Autodesk Inventor part; units mm, degrees
ref_plane "YZ Plane" through (0, 0, 0) normal (1, 0, 0) x (0, 1, 0)
ref_plane "XZ Plane" through (0, 0, 0) normal (0, 1, 0) x (-1, 0, 0)
ref_plane "XY Plane" through (0, 0, 0) normal (0, 0, 1) x (1, 0, 0)
sketch "Sketch1" plane through (0, 0, 0) normal (0, 0, 1) x (1, 0, 0)
  line L0 (-110, 70) -> (110, 70) construction
  line L1 (110, 70) -> (110, -70) construction
  line L2 (110, -70) -> (-110, -70) construction
  line L3 (-110, -70) -> (-110, 70) construction
  circle A0 centre (-90, 55) radius 5
  circle A1 centre (-90, -55) radius 5
  circle A2 centre (90, -55) radius 5
  circle A3 centre (-10, 45) radius 5
  line L4 (-67, 0) -> (-42, 0) construction
  line L5 (-42, 0) -> (-42, -30) construction
  line L6 (-42, -30) -> (-67, -30) construction
  line L7 (-67, -30) -> (-67, 0) construction
  circle A4 centre (-54.5, -11) radius 10 construction
  circle A5 centre (-63.5044, -24.4163) radius 3 construction
  circle A6 centre (-57.3559, -26.4695) radius 3 construction
  circle A7 centre (-51.263, -24.6531) radius 3 construction
  circle A8 centre (-45.3418, -26.5938) radius 3 construction
  arc A9 (-80.6122, 51.5548) -> (-99.3921, 51.5667) centre (-90, 55) ccw
  arc A10 (0, 45) -> (-16.4942, 52.6043) centre (-10, 45) ccw
  arc A11 (89.2256, -64.97) -> (88.3846, -45.1313) centre (90, -55) ccw
  line L8 (-100, 55) -> (-93.7227, 20.2343) construction
  line L9 (-93.7227, 20.2343) -> (-93.7227, 2.3339) construction
  line L10 (-93.7227, 2.3339) -> (-93.7227, -15.5707) construction
  line L11 (-93.7227, -15.5707) -> (-100, -55) construction
  spline S0 degree 4 poles (-100, 55) (-93.7227, 20.2343) (-93.7227, 2.3339) (-93.7227, -15.5707) (-100, -55) knots 1 1 1 1 1 2 2 2 2 2
  line L12 (-80, 55.0121) -> (-83.1179, 37.7603) construction
  line L13 (-33.0458, 38.469) -> (-16.4942, 52.6043) construction
  spline S1 degree 3 poles (-81.8662, -0.1941) (-57.8765, 11.5233) (-33.0458, 38.469) (-16.4942, 52.6043) knots 1.047287 1.047287 1.047287 1.047287 2 2 2 2
  line L14 (66.7614, -48.6708) -> (88.3846, -45.1313) construction
  line L15 (-90, -65) -> (-39.6885, -60.8902) construction
  line L16 (-39.6885, -60.8902) -> (0, -60.8902) construction
  line L17 (0, -60.8902) -> (36.6975, -60.8902) construction
  line L18 (36.6975, -60.8902) -> (89.2256, -64.97) construction
  spline S2 degree 4 poles (-90, -65) (-39.6885, -60.8902) (0, -60.8902) (36.6975, -60.8902) (89.2256, -64.97) knots 1 1 1 1 1 2 2 2 2 2
  spline S3 degree 3 poles (-13.6002, 30.0827) (-5.3402, 7.268) (-5.6398, -29.8026) (-10.5938, -50.667) knots 1.109736 1.109736 1.109736 1.109736 1.972131 1.972131 1.972131 1.972131
  line L19 (0, 45) -> (0, 17.1156) construction
  spline S4 degree 3 poles (0, 45) (0, 17.1156) (4.0635, -28.5965) (11.4843, -50.8799) knots 1 1 1 1 1.973632 1.973632 1.973632 1.973632
  arc A12 (-99.5185, -51.9345) -> (-88.3922, -64.8699) centre (-90, -55) ccw
  spline S5 degree 3 poles (-82.1602, -33.4696) (-73.7302, -5.1617) (-50.5606, 15.5541) (-16.7734, 31.5924) knots 1.116691 1.116691 1.116691 1.116691 1.939936 1.939936 1.939936 1.939936
  line L20 (-82.1602, -33.4696) -> (-73.7302, -5.1617) construction
  spline S6 degree 4 poles (-80, 55.0121) (-83.1179, 37.7603) (-84.6762, 24.5857) (-85.4554, 13.4176) (-85.4634, 2.054) knots 1 1 1 1 1 1.500456 1.500456 1.500456 1.500456 1.500456
  spline S7 degree 4 poles (-82.1602, -33.4696) (-82.7141, -35.9408) (-82.3572, -38.6467) (-81.9633, -41.4647) (-81.5291, -44.4067) knots 1.850189 1.850189 1.850189 1.850189 1.850189 1.936877 1.936877 1.936877 1.936877 1.936877
  line L21 (-82.1602, -33.4696) -> (-82.7141, -35.9408) construction
  spline S8 degree 4 poles (-79.5204, -46.4981) (-59.8812, -49.3583) (-42.9543, -51.1251) (-27.6277, -52.1691) (-12.9522, -52.5883) knots 1.043038 1.043038 1.043038 1.043038 1.043038 1.405573 1.405573 1.405573 1.405573 1.405573
  spline S9 degree 4 poles (13.9278, -52.5889) (30.7931, -52.1056) (47.9331, -50.8127) (66.7614, -48.6708) (88.3846, -45.1313) knots 1.574481 1.574481 1.574481 1.574481 1.574481 2 2 2 2 2
  arc A13 (-13.6002, 30.0827) -> (-16.7734, 31.5924) centre (-15.9509, 29.2316) ccw
  line L22 (-73.7302, -5.1617) -> (-50.5606, 15.5541) construction
  line L23 (-50.5606, 15.5541) -> (-16.7734, 31.5924) construction
  line L24 (-13.6002, 30.0827) -> (-5.3402, 7.268) construction
  arc A14 (-13.2443, -52.5799) -> (-10.5938, -50.667) centre (-13.0262, -50.0894) ccw
  line L25 (-5.3402, 7.268) -> (-5.6398, -29.8026) construction
  line L26 (-5.6398, -29.8026) -> (-10.5938, -50.667) construction
  line L27 (-27.6277, -52.1691) -> (-12.9522, -52.5883) construction
  arc A15 (11.4843, -50.8799) -> (13.9278, -52.5889) centre (13.8562, -50.09) ccw
  line L28 (0, 17.1156) -> (4.0635, -28.5965) construction
  line L29 (4.0635, -28.5965) -> (11.4843, -50.8799) construction
  line L30 (13.9278, -52.5889) -> (30.7931, -52.1056) construction
  line L31 (30.7931, -52.1056) -> (47.9331, -50.8127) construction
  line L32 (47.9331, -50.8127) -> (66.7614, -48.6708) construction
  arc A16 (-81.5291, -44.4067) -> (-79.5204, -46.4981) centre (-79.0558, -44.0416) ccw
  line L33 (-82.7141, -35.9408) -> (-82.3572, -38.6467) construction
  line L34 (-82.3572, -38.6467) -> (-81.9633, -41.4647) construction
  line L35 (-81.9633, -41.4647) -> (-81.5291, -44.4067) construction
  line L36 (-79.5204, -46.4981) -> (-59.8812, -49.3583) construction
  line L37 (-59.8812, -49.3583) -> (-42.9543, -51.1251) construction
  line L38 (-42.9543, -51.1251) -> (-27.6277, -52.1691) construction
  arc A17 (-85.4634, 2.054) -> (-81.8662, -0.1941) centre (-82.9634, 2.0522) ccw
  line L39 (-83.1179, 37.7603) -> (-84.6762, 24.5857) construction
  line L40 (-84.6762, 24.5857) -> (-85.4554, 13.4176) construction
  line L41 (-85.4554, 13.4176) -> (-85.4634, 2.054) construction
  line L42 (-81.8662, -0.1941) -> (-57.8765, 11.5233) construction
  line L43 (-57.8765, 11.5233) -> (-33.0458, 38.469) construction
  point P0 (0, 0)
  dimension "d1" = 70
  dimension "d2" = 70
  dimension "d3" = 110
  dimension "d4" = 110
  dimension "d5" = 10
  dimension "d6" = 10
  dimension "d7" = 10
  dimension "d8" = 10
  dimension "d9" = 55
  dimension "d10" = 55
  dimension "d11" = 55
  dimension "d12" = 180
  dimension "d13" = 90
  dimension "d14" = 90
  dimension "d15" = 10
  dimension "d16" = 45
  dimension "d17" = 42
  dimension "d18" = 30
  dimension "d19" = 0
  dimension "d20" = 25
  dimension "d21" = 20
  dimension "d22" = 6
  dimension "d23" = 6
  dimension "d24" = 6
  dimension "d25" = 11
  dimension "d26" = 12.5
  dimension "d27" = 6
  dimension "d28" = 20
  dimension "d29" = 20
  dimension "d30" = 20
  dimension "d34" = 5
  dimension "d35" = 5
  dimension "d36" = 5
  dimension "d37" = 5
  dimension "d38" = 5
extrude "Extrusion2" add sketch "Sketch1" along normal blind 9.5 contours S6 A17 S1 A10 S4 A15 S9 A11 S2 A12 S0 A9
equation "\"d26\" = 0.5 * d20"
properties part number "Bracket Concept MK1"
Here's how the part is built. I have some questions about the finished solid (model axes, mm). A direction names the side the tool comes from. Give positions to 0.01 mm unless a question says otherwise; leave off trailing zeros. One line per item, written item: value. Start each with the question number.
1. I need wall thicknesses on probe 1 along Y at (x, z) = (-90, 2.25); probe 2 along X at (y, z) = (40.5, 3.75); probe 3 along Y at (x, z) = (90, 3.75). Which ranges of each line are inside material? Lowest first, please. Write a range as from..to.
2. Will these pins go through, and if not, where does the flat tip stop? pin 1 Ø5 at (y, z) = (48, 6) entering from +X; pin 2 Ø5 at (y, z) = (7.5, 4) entering from +X; pin 3 Ø5 at (x, z) = (-76.5, 6) entering from -Y.
3. We'd pull the mould along Y, two halves only. Please class faces 3 (the face through (-7, 41, 5)), 4 (the face through (0, -14, 0)), 5 (the face through (-90, 65, 5)): released by +Y, released by -Y, zero draft, split by the parting line, or undercut.
4. Imagine slicing it at A-A, the plane y = 17.5. Count the separate pieces of the cut face and the enclosed holes in it, plus the area to 3 significant figures.
5. For faces 1 (the face through (-96.99, -62.15, 4.68)), 2 (the face through (-84.258, -0.086, 4.684)), which set-ups out of +Z, -Z, +X, -X, +Y, -Y let a thin tool reach every point of the face, with its end or its side?
Values follow:
1. probe 1: y = -65..-60, -50..50, 60..65
1. probe 2: x = -97.61..-82.38, -29.82..-12.18, -7.82..0.03
1. probe 3: y = -65..-60, -50..-45
2. pin 1: stops at x = -0.01
2. pin 2: stops at x = 1.96
2. pin 3: stops at y = -64.16
3. face 3: undercut
3. face 4: zero draft
3. face 5: released by +Y
4. separate pieces: 3
4. enclosed holes: 0
4. area: 333 mm2
5. face 1: +Z, -Z, -X, -Y
5. face 2: +Z, -Z
